The model under review builds one solid part; all positions refer to its coordinate system, in mm. Give positions to 0.01 mm unless a question says otherwise; leave off trailing zeros. Order: outer loops, then holes, each group sorted by start corner. A loop starts at its lowest first (then second) coordinate and runs counter-clockwise, first axis right, second up.
```python
from build123d import *

# Parameters (mm, degrees)
SKETCH1_W           = 13.5
SKETCH1_H           = 20
BOSS_EXTRUDE1_DEPTH = 1.5
SKETCH2_W           = 4
SKETCH2_H           = 4
BOSS_EXTRUDE2_DEPTH = 1.5
SKETCH3_R           = 0.75
CUT_EXTRUDE1_DEPTH  = 1.5
SKETCH4_W           = 8.5
SKETCH4_H           = 2
BOSS_EXTRUDE3_DEPTH = 1.5
SKETCH5_W           = 19
SKETCH5_H           = 28
SKETCH5_W_2         = 13.5
SKETCH5_H_2         = 20
BOSS_EXTRUDE4_DEPTH = 1.5


with BuildPart() as part:
    # Sketch1 → Boss-Extrude1 (new body)
    with BuildSketch(Plane(origin=(0, 0, 0), x_dir=(1, 0, 0), z_dir=(0, 1, 0))):
        with Locations((6.75, 10)):
            Rectangle(SKETCH1_W, SKETCH1_H)
    extrude(amount=BOSS_EXTRUDE1_DEPTH)

    # Sketch2 → Boss-Extrude2 (add)
    with BuildSketch(Plane(origin=(0, 1.5, 0), x_dir=(1, 0, 0), z_dir=(0, 1, 0))):
        with Locations((6.75, 15.8)):
            Rectangle(SKETCH2_W, SKETCH2_H)
        Polygon((4.5, 11.87318686), (9, 11.87318686), (9.75, 10.87318686), (3.75, 10.87318686), align=None)
    extrude(amount=BOSS_EXTRUDE2_DEPTH)

    # Sketch3 → Cut-Extrude1 (cut)
    with BuildSketch(Plane.XZ):
        with Locations(Location((12.3, -18.8, 0), (0, 0, 270))):
            Circle(SKETCH3_R)
        with Locations(Location((1.2, -1.2, 0), (0, 0, 270))):
            Circle(SKETCH3_R)
    extrude(amount=-CUT_EXTRUDE1_DEPTH, mode=Mode.SUBTRACT)

    # Sketch4 → Boss-Extrude3 (add)
    with BuildSketch(Plane(origin=(0, 1.5, 0), x_dir=(1, 0, 0), z_dir=(0, 1, 0))):
        with Locations((7.05, 1)):
            Rectangle(SKETCH4_W, SKETCH4_H)
    extrude(amount=BOSS_EXTRUDE3_DEPTH)

    # Sketch5 → Boss-Extrude4 (add)
    with BuildSketch(Plane(origin=(0, 1.5, 0), x_dir=(1, 0, 0), z_dir=(0, 1, 0))):
        with Locations((6.75, 9)):
            Rectangle(SKETCH5_W, SKETCH5_H)
        with Locations((6.75, 10)):
            Rectangle(SKETCH5_W_2, SKETCH5_H_2, mode=Mode.SUBTRACT)
    extrude(amount=-BOSS_EXTRUDE4_DEPTH)


solid = part.part
```
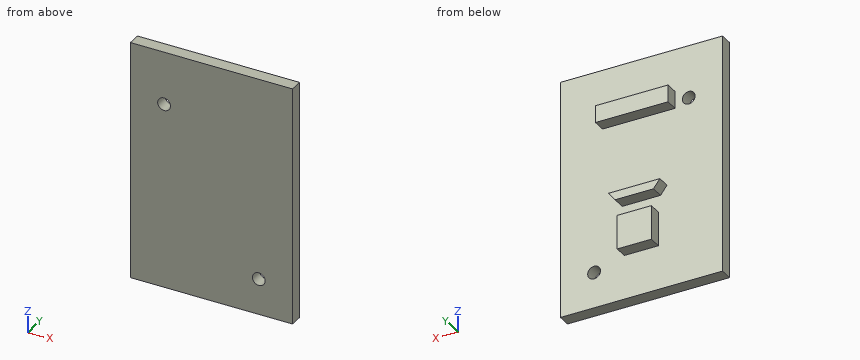
1. Insertion check: pin 1 (1.2 mm diameter, centred on x = 8, y = 2.5, fed in from +Z); pin 2 (1.2 mm diameter, centred on x = 6, y = 2.5, fed in from -Z); pin 3 (2 mm diameter, centred on x = 12.3, z = -18.8, fed in from +Y). Each pin has a flat end and moves straight along its axis. Give the tip position at first contact, or say it passes through.
2. Take a section at A-A (y = 2.05). Write out the cut boundary in (x, z).
3. Take a section at C-C (z = -18.8). Write out the cut boundary in (x, y), and give its area (4 significant figures).
4. Take a section at B-B (x = 1.2). Write out the cut boundary in (y, z).
5. To check wall thickness, follow line 1 (Z direction, x = 5.75, y = 2.75); line 2 (X direction, y = 0.55, z = -18.8); line 3 (X direction, y = 0.7, z = -1.2). State the ranges of each line that lie inside material, in increasing order.
6. Take a section at D-D (x = 10.75). Write out the cut boundary in (y, z), and give its area (3 significant figures).
Answer:
1. pin 1: stops at z = 0
1. pin 2: stops at z = -17.8
1. pin 3: stops at y = 1.5
2. outline: (2.8, -2) - (11.3, -2) - (11.3, 0) - (2.8, 0) - close; (3.75, -10.87) - (4.5, -11.87) - (9, -11.87) - (9.75, -10.87) - close; (4.75, -17.8) - (8.75, -17.8) - (8.75, -13.8) - (4.75, -13.8) - close
3. outline: (-2.75, 0) - (11.55, 0) - (11.55, 1.5) - (-2.75, 1.5) - close; (13.05, 0) - (16.25, 0) - (16.25, 1.5) - (13.05, 1.5) - close
3. area: 26.25 mm2
4. outline: (0, -23) - (1.5, -23) - (1.5, -1.95) - (0, -1.95) - close; (0, -0.45) - (1.5, -0.45) - (1.5, 5) - (0, 5) - close
5. line 1: z = -17.8 to -13.8, -11.87 to -10.87, -2 to 0
5. line 2: x = -2.75 to 11.55, 13.05 to 16.25
5. line 3: x = -2.75 to 0.45, 1.95 to 16.25
6. outline: (0, -23) - (1.5, -23) - (1.5, -2) - (3, -2) - (3, 0) - (1.5, 0) - (1.5, 5) - (0, 5) - close
6. area: 45.0 mm2
